Read the model definition and answer for the solid it produces. Units are mm, in the model's axes. A direction names the side the tool comes from. Give positions to 0.01 mm unless a question says otherwise; leave off trailing zeros. Loops run counter-clockwise (first coordinate to the right, second up) from the corner with the lowest first, then second, coordinate; pieces in that order, holes last. Notation, with made-up numbers: (75, -4) - (111, -4) arc R11 cw to (111, 2) - close; hole circle Ø9 at (-23.5, 25.25). An arc over 180 degrees is marked (long way). Put each result on its own line as item: value. Start each with the question number.
1. Consider L1, parallel to X at y = -2.75, z = 1; L2, parallel to Y at x = 40.5, z = 1.25; L3, parallel to Y at x = 4, z = 1.7. Determine where each line is inside the solid, lowest interval first. Write a range as from..to.
2. For a pull along Y with two mould halves and no side action, classify faces 3 (the flat face through (-1, 9, 1)), 4 (the flat face through (-18.3, 0, 1)), 5 (the flat face through (18.3, 0, 1)), 6 (the flat face through (-1, 0, 0)) as released by +Y, released by -Y, zero draft, split by the parting line, or undercut.
3. A cutting plane is placed at C-C, the plane x = -4. Determine the outline of the cut face in (y, z), plus the area to 3 significant figures.
4. A cutting plane is placed at B-B, the plane z = 1.3. Determine the outline of the cut face in (x, y).
5. For faces 1 (the flat face through (-65, 0, 1)), 2 (the flat face through (-39.9, 0, 1)), determine the directions among +Z, -Z, +X, -X, +Y, -Y from which every point of the face is accessible in a straight line to the end or side of a thin tool.
6. A cutting plane is placed at A-A, the plane y = 0.25. Determine the outline of the cut face in (x, z), plus the area to 3 significant figures.
```python
from build123d import *

# Parameters (mm, degrees)
SKETCH2_W           = 130
SKETCH2_H           = 18
BOSS_EXTRUDE1_DEPTH = 2.4
SKETCH3_W           = 1.8
SKETCH3_H           = 11
SKETCH3_H_2         = 5.5
CUT_EXTRUDE1_DEPTH  = 11


with BuildPart() as part:
    # Sketch2 → Boss-Extrude1 (new body)
    with BuildSketch(Plane.XY):
        Rectangle(SKETCH2_W, SKETCH2_H)
    extrude(amount=BOSS_EXTRUDE1_DEPTH)

    # Sketch3 → Cut-Extrude1 (cut)
    with BuildSketch(Plane.XY.offset(2.4)):
        with Locations((-40.8, 0)):
            Rectangle(SKETCH3_W, SKETCH3_H)
        with Locations((-19.2, 2.75)):
            Rectangle(SKETCH3_W, SKETCH3_H_2)
        with Locations((-19.2, -2.75)):
            Rectangle(SKETCH3_W, SKETCH3_H_2)
        with Locations((19.2, 0)):
            Rectangle(SKETCH3_W, SKETCH3_H)
        with Locations((40.8, 0)):
            Rectangle(SKETCH3_W, SKETCH3_H)
        Polygon((0, 3), (0, 3.9), (-5.5, 3.9), (-5.5, 2.1), (0, 2.1), align=None)
        Polygon((5.5, 3.9), (0, 3.9), (0, 3), (0, 2.1), (5.5, 2.1), align=None)
    extrude(amount=-CUT_EXTRUDE1_DEPTH, mode=Mode.SUBTRACT)


solid = part.part
```
Return value:
1. L1: x = -65..-41.7, -39.9..-20.1, -18.3..18.3, 20.1..39.9, 41.7..65
1. L2: y = -9..-5.5, 5.5..9
1. L3: y = -9..2.1, 3.9..9
2. face 3: released by +Y
2. face 4: undercut
2. face 5: undercut
2. face 6: zero draft
3. outline: (-9, 0) - (2.1, 0) - (2.1, 2.4) - (-9, 2.4) - close; (3.9, 0) - (9, 0) - (9, 2.4) - (3.9, 2.4) - close
3. area: 38.9 mm2
4. outline: (-65, -9) - (65, -9) - (65, 9) - (-65, 9) - close; hole (-41.7, -5.5) - (-39.9, -5.5) - (-39.9, 5.5) - (-41.7, 5.5) - close; hole (-20.1, -5.5) - (-18.3, -5.5) - (-18.3, 5.5) - (-20.1, 5.5) - close; hole (-5.5, 2.1) - (5.5, 2.1) - (5.5, 3.9) - (-5.5, 3.9) - close; hole (18.3, -5.5) - (20.1, -5.5) - (20.1, 5.5) - (18.3, 5.5) - close; hole (39.9, -5.5) - (41.7, -5.5) - (41.7, 5.5) - (39.9, 5.5) - close
5. face 1: +Z, -Z, -X, +Y, -Y
5. face 2: +Z, -Z
6. outline: (-65, 0) - (-41.7, 0) - (-41.7, 2.4) - (-65, 2.4) - close; (-39.9, 0) - (-20.1, 0) - (-20.1, 2.4) - (-39.9, 2.4) - close; (-18.3, 0) - (18.3, 0) - (18.3, 2.4) - (-18.3, 2.4) - close; (20.1, 0) - (39.9, 0) - (39.9, 2.4) - (20.1, 2.4) - close; (41.7, 0) - (65, 0) - (65, 2.4) - (41.7, 2.4) - close
6. area: 295 mm2
